from build123d import *

# Parameters (mm, degrees)
BOSS_EXTRUDE1_DEPTH = 4
SKETCH2_R           = 2
CUT_EXTRUDE1_DEPTH  = 4
SKETCH3_R           = 2
CUT_EXTRUDE2_DEPTH  = 4
SKETCH4_R           = 2
CUT_EXTRUDE3_DEPTH  = 4
SKETCH5_W           = 2
SKETCH5_H           = 90
BOSS_EXTRUDE2_DEPTH = 4
SKETCH6_R           = 2
CUT_EXTRUDE4_DEPTH  = 4
SKETCH7_R           = 11.5
CUT_EXTRUDE5_DEPTH  = 10


with BuildPart() as part:
    # Sketch1 → Boss-Extrude1 (new body)
    with BuildSketch(Plane.XY):
        Polygon((-45, 27), (-45, 63), (0, 63), (0, 27), (45, 27), (45, -27), (-45, -27), align=None)
    extrude(amount=BOSS_EXTRUDE1_DEPTH)

    # Sketch2 → Cut-Extrude1 (cut)
    with BuildSketch(Plane.XY.offset(4)):
        with Locations((-40.5, -22.5)):
            Circle(SKETCH2_R)
        with Locations((-30.5, -22.5)):
            Circle(SKETCH2_R)
        with Locations(Location((30.5, -22.5, 0), (0, 0, 180))):
            Circle(SKETCH2_R)
        with Locations(Location((40.5, -22.5, 0), (0, 0, 180))):
            Circle(SKETCH2_R)
        with Locations(Location((30.5, 22.5, 0), (0, 0, 180))):
            Circle(SKETCH2_R)
        with Locations(Location((40.5, 22.5, 0), (0, 0, 180))):
            Circle(SKETCH2_R)
    extrude(amount=-CUT_EXTRUDE1_DEPTH, mode=Mode.SUBTRACT)

    # Sketch3 → Cut-Extrude2 (cut)
    with BuildSketch(Plane.XY.offset(4)):
        with Locations((-40.5, 24.080850084)):
            Circle(SKETCH3_R)
        with Locations((-9.500034607, 24.034529107)):
            Circle(SKETCH3_R)
    extrude(amount=-CUT_EXTRUDE2_DEPTH, mode=Mode.SUBTRACT)

    # Sketch4 → Cut-Extrude3 (cut)
    with BuildSketch(Plane.XY.offset(4)):
        with Locations((-40.690838772, 55.080850084)):
            Circle(SKETCH4_R)
        with Locations((-9.690838772, 55.080850084)):
            Circle(SKETCH4_R)
    extrude(amount=-CUT_EXTRUDE3_DEPTH, mode=Mode.SUBTRACT)

    # Sketch5 → Boss-Extrude2 (add)
    with BuildSketch(Plane.XY.offset(4)):
        with Locations((-46, 18)):
            Rectangle(SKETCH5_W, SKETCH5_H)
    extrude(amount=-BOSS_EXTRUDE2_DEPTH)

    # Sketch6 → Cut-Extrude4 (cut)
    with BuildSketch(Plane.XY.offset(4)):
        with Locations((4.5, 22.5)):
            Circle(SKETCH6_R)
        with Locations((14.5, 22.5)):
            Circle(SKETCH6_R)
    extrude(amount=-CUT_EXTRUDE4_DEPTH, mode=Mode.SUBTRACT)

    # Sketch7 → Cut-Extrude5 (cut)
    with BuildSketch(Plane.XY.offset(4)):
        with Locations((-25.09543669, 39.557689595)):
            Circle(SKETCH7_R)
    extrude(amount=-CUT_EXTRUDE5_DEPTH, mode=Mode.SUBTRACT)


solid = part.part
Source: CAD feature listing. Evaluate the final solid. Frame: model axes, mm. A direction names the side the tool comes from. Round coordinates to 2 decimals unless told otherwise and drop trailing zeros. Loops run counter-clockwise (first coordinate to the right, second up) from the corner with the lowest first, then second, coordinate; pieces in that order, holes last. Notation, with made-up numbers: (-20, 20) - (6, 20) arc R28 cw to (6, 49) - close; hole circle Ø10 at (-28.75, 10.5). An arc over 180 degrees is marked (long way). Write item = value, one per line. Start each with the question number.
(1) Pull-direction query (Y, two-part tool) for faces 3 (the face through (-24, 63, 2)), 4 (the face through (-2, -27, 2)), 5 (the face through (-12, 9, 4)), 6 (the face through (28.592, -23.101, 2.028)); classes: +Y half, -Y half, draft (parallel to the pull), parting line (faces both ways), or undercut.
(2) Section query B-B, the plane y = -22.5. Output: boundary loops of the cut face in (x, z).
(3) Pin query (flat end, axial travel): pin 1 (1.2 mm diameter, centred on y = 39.5, z = 1, fed in from +X); pin 2 (1.2 mm diameter, centred on x = 20, z = 1, fed in from +Y). Return the tip coordinate at first contact, or that it passes through.
(4) Section query D-D, the plane x = -40.5. Output: boundary loops of the cut face in (y, z).
(5) Section query A-A, the plane x = 4.5. Output: boundary loops of the cut face in (y, z).
(6) Ray query, line 1 along Y through (x, z) = (30.5, 2.4); line 2 along Y through (x, z) = (-40.5, 2.6); line 3 along Y through (x, z) = (29, 1.8). Return the intervals inside material, ascending. Write a range as from..to.
(7) Section query C-C, the plane x = 40.5. Output: boundary loops of the cut face in (y, z), plus the area to 3 significant figures.
(8) Set-up query: faces 1 (the face through (28.592, 21.899, 2.028)), 2 (the face through (0, 45, 2)). Return all of +Z, -Z, +X, -X, +Y, -Y with unobstructed straight access to the full face (end or side cutting, diameter ignored); none if empty.
Conclusion:
q1.face_3 = +Y half
q1.face_4 = -Y half
q1.face_5 = draft
q1.face_6 = undercut
q2.outline = (-47, 0) - (-42.5, 0) - (-42.5, 4) - (-47, 4) - close; (-38.5, 0) - (-32.5, 0) - (-32.5, 4) - (-38.5, 4) - close; (-28.5, 0) - (28.5, 0) - (28.5, 4) - (-28.5, 4) - close; (32.5, 0) - (38.5, 0) - (38.5, 4) - (32.5, 4) - close; (42.5, 0) - (45, 0) - (45, 4) - (42.5, 4) - close
q3.pin_1 = 0
q3.pin_2 = 27
q4.outline = (-27, 0) - (-24.5, 0) - (-24.5, 4) - (-27, 4) - close; (-20.5, 0) - (22.08, 0) - (22.08, 4) - (-20.5, 4) - close; (26.08, 0) - (53.09, 0) - (53.09, 4) - (26.08, 4) - close; (57.07, 0) - (63, 0) - (63, 4) - (57.07, 4) - close
q5.outline = (-27, 0) - (20.5, 0) - (20.5, 4) - (-27, 4) - close; (24.5, 0) - (27, 0) - (27, 4) - (24.5, 4) - close
q6.line_1 = -27..-24.5, -20.5..20.5, 24.5..27
q6.line_2 = -27..-24.5, -20.5..22.08, 26.08..53.09, 57.07..63
q6.line_3 = -27..-23.82, -21.18..21.18, 23.82..27
q7.outline = (-27, 0) - (-24.5, 0) - (-24.5, 4) - (-27, 4) - close; (-20.5, 0) - (20.5, 0) - (20.5, 4) - (-20.5, 4) - close; (24.5, 0) - (27, 0) - (27, 4) - (24.5, 4) - close
q7.area = 184 mm2
q8.face_1 = +Z, -Z
q8.face_2 = +Z, -Z, +X, +Y
